from build123d import *

# Parameters (mm, degrees)
PAD001_DEPTH    = 102.5
POCKET002_DEPTH = 10
SKETCH007_R     = 1.6
POCKET005_DEPTH = 5
SKETCH008_R     = 8.2
POCKET006_DEPTH = 2.5
SKETCH026_R     = 6.5
PAD010_DEPTH    = 3
SKETCH027_R     = 6.5
PAD011_DEPTH    = 3


with BuildPart() as part:
    # Sketch003 → Pad001 (new body, symmetric)
    with BuildSketch(Plane.XZ):
        Polygon((0, 0), (35, 0), (35, 2), (3, 2), (3, 20), (5, 22), (5, 31), (10, 36), (10, 48), (0, 48), align=None)
    extrude(amount=PAD001_DEPTH, both=True)

    # Sketch004 (on Face9 of Pad001) → Pocket002 (cut)
    with BuildSketch(Plane(origin=(0, 0, 48), x_dir=(-1, 0, 0), z_dir=(0, 0, 1))):
        Polygon((-10, 98.5), (-7, 98.5), (-7, 100.5), (-3.4, 100.5), (-3.4, 98.5), (0, 98.5), (0, 78.5), (-3.4, 78.5), (-3.4, -78.5), (0, -78.5), (0, -98.5), (-3.4, -98.5), (-3.4, -100.5), (-7, -100.5), (-7, -98.5), (-10, -98.5), align=None)
    extrude(amount=-POCKET002_DEPTH, mode=Mode.SUBTRACT)

    # Sketch007 (on Face17 of Pocket002) → Pocket005 (cut)
    with BuildSketch(Plane(origin=(5, 0, 0), x_dir=(0, 0, 1), z_dir=(1, 0, 0))):
        with Locations((26.5, 0)):
            Circle(SKETCH007_R)
    extrude(amount=-POCKET005_DEPTH, mode=Mode.SUBTRACT)

    # Sketch008 → Pocket006 (cut, symmetric)
    with BuildSketch(Plane.XY):
        with Locations((17.5, 0)):
            Circle(SKETCH008_R)
        with Locations((17.5, 64)):
            Circle(SKETCH008_R)
        with Locations((17.5, 32)):
            Circle(SKETCH008_R)
        with Locations((17.5, -32)):
            Circle(SKETCH008_R)
        with Locations((17.5, -64)):
            Circle(SKETCH008_R)
    extrude(amount=POCKET006_DEPTH, both=True, mode=Mode.SUBTRACT)

    # Sketch026 (on Face3 of Pocket006) → Pad010 (join)
    with BuildSketch(Plane(origin=(0, 102.5, 0), x_dir=(1, 0, 0), z_dir=(0, 1, 0))):
        Polygon((0, -36), (0, 0), (35, 0), (35, -2), (10, -36), align=None)
        with Locations((10, -9)):
            Circle(SKETCH026_R, mode=Mode.SUBTRACT)
    extrude(amount=-PAD010_DEPTH)

    # Sketch027 (on Face1 of Pad010) → Pad011 (join)
    with BuildSketch(Plane.XZ.offset(102.5)):
        Polygon((35, 2), (10, 36), (0, 36), (0, 0), (35, 0), align=None)
        with Locations((10, 9)):
            Circle(SKETCH027_R, mode=Mode.SUBTRACT)
    extrude(amount=-PAD011_DEPTH)


with BuildPart() as part_1:
    # Body001 placement: moved
    add(part.part.moved(Location((50, -150, 0))))


solid = part_1.part
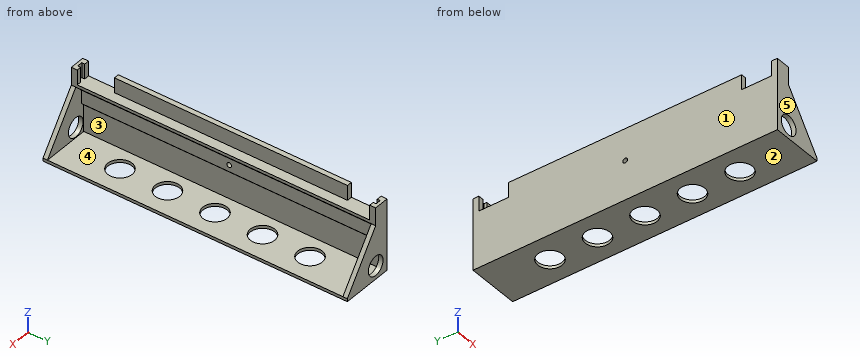
Part model, mm, in its own coordinate system. Face numbers are marked on the shaded views. A direction names the side the tool comes from. Coordinates: 2 decimals unless noted, no trailing zeros. Loops run counter-clockwise (first coordinate to the right, second up) from the corner with the lowest first, then second, coordinate; pieces in that order, holes last. Notation, with made-up numbers: M -35.5,20 L -20.5,20 A14 cw -20.5,33 Z; hole C -10,-25 d3. An arc over 180 degrees is marked long. Use a Markdown table: item, result. Add a question column.
Q1. Cut at B-B (z = 43). Write the cut outline in (x, y), and give its area (3 significant figures).
Q2. Cut at C-C (x = 78). Write the cut outline in (y, z), and give its area (3 significant figures).
Q3. Cut at A-A (y = -214). Write the cut outline in (x, z).
Q4. Pin check, flat tips, straight feed: P1, Ø10, axis at x = 75, y = -157.5, coming from the +Z side; P2, Ø1, axis at y = -50.5, z = 42.5, coming from the +X side; P3, Ø6, axis at y = -204.5, z = 19.5, coming from the +X side. Stop position of each tip, or through.
Q5. Cut at D-D (z = 9). Write the cut outline in (x, y), and give its area (3 significant figures).
Q6. Mould opens along Z. For the marked faces 1, 2 and 3 say: +Z half, -Z half, draft (parallel to the pull), parting line (faces both ways), or undercut.
Q7. Probe L1, parallel to Y at x = 58, z = 23.5; L2, parallel to X at y = -86, z = 0.8; L3, parallel to Z at x = 73.5, y = -167. List the from-to ranges inside material, lowest first.
Q8. Which spindle directions (+Z, -Z, +X, -X, +Y, -Y) get a long thin tool onto all of the face, cutting with end or side? Do the marked faces 4 and 5. Say none if no direction does.
Worked out:
| question | item | result |
|---|---|---|
| 1 | outline | M 50,-252.5 L 60,-252.5 L 60,-248.5 L 57,-248.5 L 57,-250.5 L 53.4,-250.5 L 53.4,-248.5 L 50,-248.5 Z; M 50,-228.5 L 53.4,-228.5 L 53.4,-71.5 L 50,-71.5 Z; M 50,-51.5 L 53.4,-51.5 L 53.4,-49.5 L 57,-49.5 L 57,-51.5 L 60,-51.5 L 60,-47.5 L 50,-47.5 Z |
| 1 | area | 599 mm2 |
| 2 | outline | M -252.5,0 L -47.5,0 L -47.5,11.52 L -50.5,11.52 L -50.5,2 L -249.5,2 L -249.5,11.52 L -252.5,11.52 Z |
| 2 | area | 467 mm2 |
| 3 | outline | M 50,0 L 59.3,0 L 59.3,2 L 53,2 L 53,20 L 55,22 L 55,31 L 60,36 L 60,38 L 53.4,38 L 53.4,48 L 50,48 Z; M 75.7,0 L 85,0 L 85,2 L 75.7,2 Z |
| 4 | P1 | stops at z = 2 |
| 4 | P2 | stops at x = 60 |
| 4 | P3 | stops at x = 55 |
| 5 | outline | M 50,-252.5 L 53.5,-252.5 L 53.5,-249.5 L 53,-249.5 L 53,-50.5 L 53.5,-50.5 L 53.5,-47.5 L 50,-47.5 Z; M 66.5,-252.5 L 79.85,-252.5 L 79.85,-249.5 L 66.5,-249.5 Z; M 66.5,-50.5 L 79.85,-50.5 L 79.85,-47.5 L 66.5,-47.5 Z |
| 5 | area | 698 mm2 |
| 6 | face 1 | draft |
| 6 | face 2 | -Z half |
| 6 | face 3 | undercut |
| 7 | L1 | y = -252.5 to -249.5, -50.5 to -47.5 |
| 7 | L2 | x = 50 to 59.3, 75.7 to 85 |
| 7 | L3 | z = 0 to 2 |
| 8 | face 4 | +X |
| 8 | face 5 | +Z, -Z, +X, -X, -Y |
